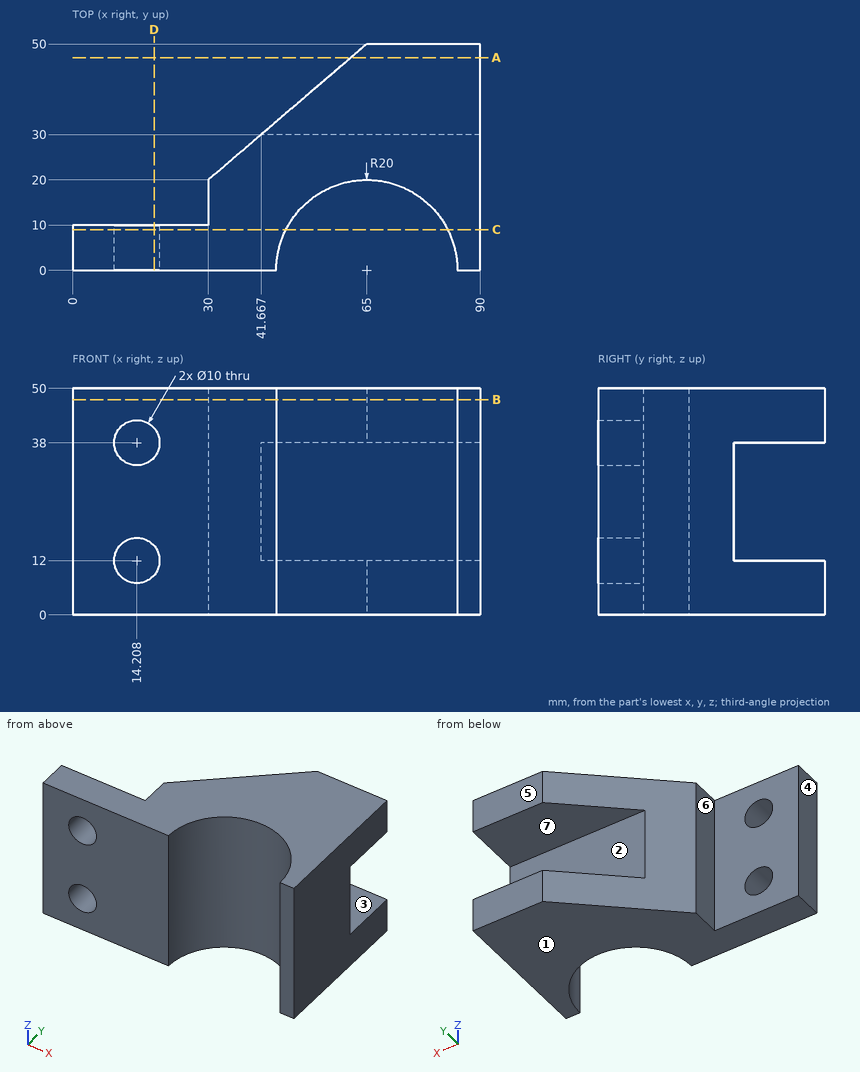
Input: dimensioned drawing with shaded views. Units: mm. Origin: part minimum x, y, z. A direction names the side the tool comes from. Give positions to 0.01 mm unless a question says otherwise; leave off trailing zeros. Write each loop counter-clockwise with the first axis right and the second up, starting at its lowest first coordinate (ties: lowest second). Pieces come first, ordered by that corner, then holes. Notation, with made-up numbers: (-40, 38) -> (-15, 38) arc R20 ccw to (-15, 74) -> close; hole circle Ø8 at (1, 77.5). An arc over 180 degrees is marked (long way). Return JSON: item names as keys, results as strings. Group by question number.
1. Mould query, pull axis Z, two halves, no side actions, for the marked faces 1, 2, 3 and 4. Classes: +Z half, -Z half, draft (parallel to the pull), parting line (faces both ways), or undercut.
2. Material intervals for line 1 (X direction, y = 3, z = 38); line 2 (X direction, y = 8, z = 12); line 3 (Z direction, x = 58.5, y = 36), sorted ascending. Write a range as from..to.
3. Access query for the marked faces 5, 6 and 7. Directions: +Z, -Z, +X, -X, +Y, -Y. A direction counts if a zero-diameter tool reaches every point of the face in a straight line with its end or side. Return the directions, or none.
4. Section D-D, the plane x = 18. Output: boundary loops of the cut face in (y, z).
5. Pin query (flat end, axial travel): pin 1 Ø9 at (x, z) = (10, 24) entering from +Y; pin 2 Ø13 at (x, z) = (69, 29) entering from +Y; pin 3 Ø4 at (y, z) = (13, 14) entering from -X. Return the tip coordinate at first contact, or that it passes through.
6. Section B-B, the plane z = 47.5. Output: boundary loops of the cut face in (x, y).
7. Section C-C, the plane y = 9. Output: boundary loops of the cut face in (x, z), then the cut area to 3 significant figures.
8. Section A-A, the plane y = 47. Output: boundary loops of the cut face in (x, z).
Determined:
{
 "1": {"face 1": "-Z half", "face 2": "undercut", "face 3": "undercut", "face 4": "draft"},
 "2": {"line 1": "x = 0..9.21, 19.21..45.23, 84.77..90", "line 2": "x = 0..9.21, 19.21..46.67, 83.33..90", "line 3": "z = 0..12, 38..50"},
 "3": {"face 5": "+Z, -Z, +X, -X, +Y", "face 6": "+Z, -Z, -X, +Y", "face 7": "+X, -X, +Y"},
 "4": {"outline": "(0, 0) -> (10, 0) -> (10, 8.74) -> (0, 8.74) -> close; (0, 15.26) -> (10, 15.26) -> (10, 34.74) -> (0, 34.74) -> close; (0, 41.26) -> (10, 41.26) -> (10, 50) -> (0, 50) -> close"},
 "5": {"pin 1": "stops at y = 10", "pin 2": "stops at y = 30", "pin 3": "stops at x = 30"},
 "6": {"outline": "(0, 0) -> (45, 0) arc R20 cw to (85, 0) -> (90, 0) -> (90, 50) -> (65, 50) -> (30, 20) -> (30, 10) -> (0, 10) -> close"},
 "7": {"outline": "(0, 0) -> (47.14, 0) -> (47.14, 50) -> (0, 50) -> close; (82.86, 0) -> (90, 0) -> (90, 50) -> (82.86, 50) -> close; hole circle Ø10 at (14.21, 12); hole circle Ø10 at (14.21, 38)", "area": "2,560 mm2"},
 "8": {"outline": "(61.5, 0) -> (90, 0) -> (90, 12) -> (61.5, 12) -> close; (61.5, 38) -> (90, 38) -> (90, 50) -> (61.5, 50) -> close"}
}
